```python
from build123d import *

# Parameters (mm, degrees)
SKETCH1_W               = 60
SKETCH1_H               = 100
BOSS_EXTRUDE1_DEPTH     = 35
SKETCH3_R               = 7.5
SKETCH3_W               = 16
SKETCH3_H               = 40
CUT_EXTRUDE1_DEPTH      = 55
CUT_EXTRUDE2_DEPTH      = 69.007352544
CUT_EXTRUDE2_DEPTH_BACK = 69.007352544
SKETCH5_R               = 4
SKETCH7_R               = 6.5
CUT_EXTRUDE3_DEPTH      = 5
CUT_EXTRUDE5_DEPTH      = 7.5


with BuildPart() as part:
    # Sketch1 → Boss-Extrude1 (new body)
    with BuildSketch(Plane.XY):
        Rectangle(SKETCH1_W, SKETCH1_H)
    extrude(amount=BOSS_EXTRUDE1_DEPTH)

    # Sketch3 → Cut-Extrude1 (cut)
    with BuildSketch(Plane(origin=(30, 0, 0), x_dir=(0, 0, -1), z_dir=(1, 0, 0))):
        with Locations((-17.5, 35)):
            Circle(SKETCH3_R)
        with Locations(Location((-17.5, -35, 0), (0, 0, 180))):
            Circle(SKETCH3_R)
        with Locations((-17.5, 0)):
            Rectangle(SKETCH3_W, SKETCH3_H)
    extrude(amount=-CUT_EXTRUDE1_DEPTH, mode=Mode.SUBTRACT)

    # Sketch5 → Cut-Extrude2 (cut, two sides: drawn at the far end of the back side and taken through both)
    with BuildSketch(Plane(origin=(0, 0, 0), x_dir=(-1, 0, 0), z_dir=(0, 0, -1)).offset(-CUT_EXTRUDE2_DEPTH_BACK)):
        Circle(SKETCH5_R)
    extrude(amount=CUT_EXTRUDE2_DEPTH + CUT_EXTRUDE2_DEPTH_BACK, mode=Mode.SUBTRACT)

    # Sketch7 → Cut-Extrude3 (cut)
    with BuildSketch(Plane.XY.offset(35)):
        Circle(SKETCH7_R)
    extrude(amount=-CUT_EXTRUDE3_DEPTH, mode=Mode.SUBTRACT)

    # Sketch8 → Cut-Extrude5 (cut)
    with BuildSketch(Plane(origin=(0, 0, 0), x_dir=(-1, 0, 0), z_dir=(0, 0, -1))):
        Polygon((0, 8.666604891), (-7.5055, 4.333302445), (-7.5055, -4.333302445), (0, -8.666604891), (7.5055, -4.333302445), (7.5055, 4.333302445), align=None)
    extrude(amount=-CUT_EXTRUDE5_DEPTH, mode=Mode.SUBTRACT)


solid = part.part
```
Check sheet for the modelled part. Datum: model origin and axes. Units: mm. A direction names the side the tool comes from. Round coordinates to 2 decimals unless told otherwise and drop trailing zeros. Order: outer loops, then holes, each group sorted by start corner. A loop starts at its lowest first (then second) coordinate and runs counter-clockwise, first axis right, second up.
1) Section check A-A (y = 0). Record the boundary of the cut face in (x, z), and give its area (3 significant figures).
2) Section check D-D (y = 35). Record the boundary of the cut face in (x, z), and give its area (4 significant figures).
3) Mould release check, pull along X, two halves, no side actions. Record for faces 5 (the cylindrical face through (0.867, -3.905, 8.514)), 6 (the flat face through (-30, -1, 17)), 7 (the flat face through (0, -50, 17)): +X half, -X half, draft (parallel to the pull), parting line (faces both ways), or undercut.
4) Section check B-B (x = -24). Record the boundary of the cut face in (y, z), and give its area (3 significant figures).
5) Go/stop test with flat-tipped pins: pin 1 Ø10.5 at (x, y) = (0, 0) entering from +Z; pin 2 Ø7.5 at (y, z) = (35.5, 21) entering from +X. Record where each tip stops, or that it passes through.
6) Scan lines: line 1 (Y direction, x = -17, z = 17); line 2 (Y direction, x = 0, z = 33.15); line 3 (Z direction, x = 22, y = 5). Record each from-to range of solid material in increasing order.
7) Section check C-C (z = 13). Record the boundary of the cut face in (x, y).
8) Tool access check on faces 1 (the flat face through (2, -4, 7.5)), 2 (the flat face through (0, 50, 17)), 3 (the flat face through (-25, 0, 18)), 4 (the cylindrical face through (-5.158, -3.955, 32.535)). Record the directions out of +Z, -Z, +X, -X, +Y, -Y that give a thin tool (end or side, any length) a straight path to the whole face; none if there is none.
Result:
1. outline: (-30, 0) - (-7.51, 0) - (-7.51, 7.5) - (-4, 7.5) - (-4, 9.5) - (-25, 9.5) - (-25, 25.5) - (-4, 25.5) - (-4, 30) - (-6.5, 30) - (-6.5, 35) - (-30, 35) - close; (4, 7.5) - (7.51, 7.5) - (7.51, 0) - (30, 0) - (30, 9.5) - (4, 9.5) - close; (4, 25.5) - (30, 25.5) - (30, 35) - (6.5, 35) - (6.5, 30) - (4, 30) - close
1. area: 990 mm2
2. outline: (-30, 0) - (30, 0) - (30, 10) - (-25, 10) - (-25, 25) - (30, 25) - (30, 35) - (-30, 35) - close
2. area: 1,275 mm2
3. face 5: undercut
3. face 6: -X half
3. face 7: draft
4. outline: (-50, 0) - (50, 0) - (50, 35) - (-50, 35) - close; hole circle Ø15 at (-35, 17.5); hole (-20, 9.5) - (20, 9.5) - (20, 25.5) - (-20, 25.5) - close; hole circle Ø15 at (35, 17.5)
4. area: 2,510 mm2
5. pin 1: stops at z = 30
5. pin 2: stops at x = -25
6. line 1: y = -50 to -42.48, -27.52 to -20, 20 to 27.52, 42.48 to 50
6. line 2: y = -50 to -6.5, 6.5 to 50
6. line 3: z = 0 to 9.5, 25.5 to 35
7. outline: (-30, -50) - (30, -50) - (30, -41) - (-25, -41) - (-25, -29) - (30, -29) - (30, -20) - (-25, -20) - (-25, 20) - (30, 20) - (30, 29) - (-25, 29) - (-25, 41) - (30, 41) - (30, 50) - (-30, 50) - close
8. face 1: -Z
8. face 2: +Z, -Z, +X, -X, +Y
8. face 3: +X
8. face 4: +Z
